Can you work these out from the drawing? Everything is in mm from the part's minimum corner. Give positions to 0.01 mm unless a question says otherwise; leave off trailing zeros. Loops run counter-clockwise (first coordinate to the right, second up) from the corner with the lowest first, then second, coordinate; pieces in that order, holes last. Notation, with made-up numbers: (83, 27) - (122, 27) arc R7 ccw to (122, 31) - close; hole circle Ø2 at (-14, 25). An arc over 180 degrees is marked (long way). Write each question's results on one line, items separated by ' | '. Start each with the question number.
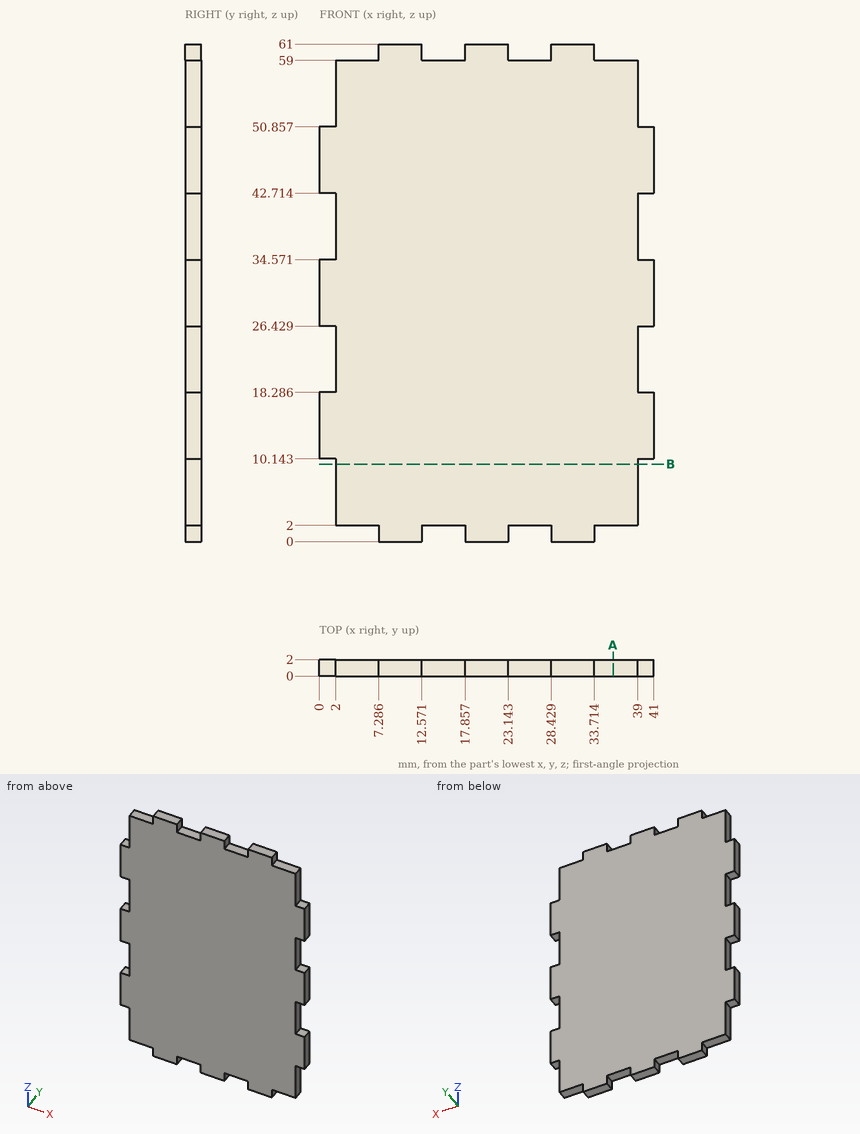
Q1. I want a section at B-B, the plane z = 9.5. List the corners of the cut face in (x, y) for me.
Q2. I'm going to push flat-ended pins straight in: pin 1 Ø0.6 at (x, y) = (16, 1) entering from +Z; pin 2 Ø1 at (y, z) = (1, 7.5) entering from -X; pin 3 Ø0.6 at (x, y) = (27, 1) entering from -Z; pin 4 Ø3 at (x, z) = (19, 31) entering from -Y. Where does each tip first touch, or does it pass through?
Q3. I need wall thicknesses on L1, parallel to Z at x = 25, y = 1.5; L2, parallel to X at y = 1.15, z = 58. Which ranges of each line are inside material? Lowest first, please. Write a range as from..to.
Q4. I want a section at A-A, the plane x = 36. List the corners of the cut face in (y, z) for me.
Conclusion:
1) outline: (2, 0) - (39, 0) - (39, 2) - (2, 2) - close
2) pin 1: z = 59 | pin 2: x = 2 | pin 3: z = 2 | pin 4: y = 0
3) L1: 2..59 | L2: 2..39
4) outline: (0, 2) - (2, 2) - (2, 59) - (0, 59) - close
